Read the model definition and answer for the solid it produces. Units are mm, in the model's axes. Face numbers are marked on the shaded views. A direction names the side the tool comes from. Give positions to 0.01 mm unless a question says otherwise; leave off trailing zeros. Order: outer loops, then holes, each group sorted by start corner. A loop starts at its lowest first (then second) coordinate and runs counter-clockwise, first axis right, second up. Notation, with made-up numbers: (13.25, 6) -> (41.25, 6) arc R8 cw to (41.25, 15) -> close; hole circle Ø5 at (36, -33.75). An arc over 180 degrees is marked (long way). One line per item, written item: value. Start each with the question number.
from build123d import *

# Parameters (mm, degrees)
SKETCH_1_W      = 32
SKETCH_1_H      = 20
SKETCH_1_R      = 1.5
EXTRUDE_1_DEPTH = 1.6
SKETCH_2_W      = 6.5
SKETCH_2_H      = 6.5
EXTRUDE_2_DEPTH = 5
SKETCH_3_R      = 9.5
EXTRUDE_3_DEPTH = 16.5


with BuildPart() as part:
    # 草图1 → 凸台-拉伸1 (new body)
    with BuildSketch(Plane(origin=(0, 0, 0), x_dir=(1, 0, 0), z_dir=(0, 1, 0))):
        Rectangle(SKETCH_1_W, SKETCH_1_H)
        with Locations(Location((-13.5, 7.5, 0), (0, 0, 270))):
            Circle(SKETCH_1_R, mode=Mode.SUBTRACT)
        with Locations(Location((13.5, 7.5, 0), (0, 0, 270))):
            Circle(SKETCH_1_R, mode=Mode.SUBTRACT)
        with Locations(Location((-13.5, -7.5, 0), (0, 0, 270))):
            Circle(SKETCH_1_R, mode=Mode.SUBTRACT)
        with Locations(Location((13.5, -7.5, 0), (0, 0, 270))):
            Circle(SKETCH_1_R, mode=Mode.SUBTRACT)
    extrude(amount=EXTRUDE_1_DEPTH)

    # 草图2 → 凸台-拉伸2 (add)
    with BuildSketch(Plane(origin=(0, 0, 0), x_dir=(1, 0, 0), z_dir=(0, 1, 0))):
        with Locations((7.75, -6.25)):
            Rectangle(SKETCH_2_W, SKETCH_2_H)
    extrude(amount=-EXTRUDE_2_DEPTH)

    # 草图3 → 凸台-拉伸3 (add)
    with BuildSketch(Plane(origin=(0, 0, 0), x_dir=(1, 0, 0), z_dir=(0, 1, 0))):
        with Locations(Location((-5, 0, 0), (0, 0, 270))):
            Circle(SKETCH_3_R)
    extrude(amount=EXTRUDE_3_DEPTH)

    # 草图4 → 切除-旋转2 (revolve, cut)
    with BuildSketch(Plane.XY):
        Polygon((-0.3, 16.5), (0.5, 16.5), (4.5, 16.5), (4.5, 6.5), (3, 6.5), (0.766666667, 15.433333333), align=None)
    revolve(axis=Axis((-5, -983.5, 0), (0, 1, 0)), mode=Mode.SUBTRACT)


solid = part.part
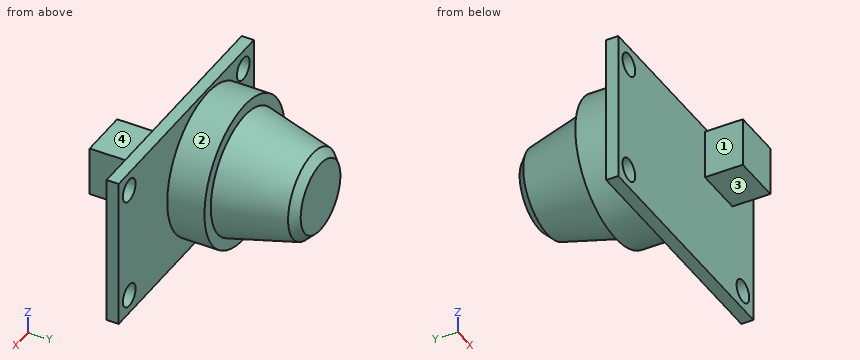
Item 1: Find section D-D on x = -5. Write down the section's boundary in (y, z).
Item 2: Find the intervals of material crossed by line 1 (X direction, y = 0.8, z = -7.5); line 2 (Z direction, x = 14, y = 1.5); line 3 (Y direction, x = -13, z = -5), in increasing order. Write a range as from..to.
Item 3: Flat-ended cylindrical pins translate along their axes: pin 1 (5 mm diameter, centred on x = 13.5, z = -7.5, fed in from -Y); pin 2 (2.5 mm diameter, centred on x = -13.5, z = 7.5, fed in from -Y); pin 3 (5.5 mm diameter, centred on y = -1.5, z = 7, fed in from -X); pin 4 (3 mm diameter, centred on x = -12.5, y = 6.5, fed in from -Z). Find the tip coordinate at first contact, or state that the pin passes through.
Item 4: Find section B-B on z = 0. Write down the section's boundary in (x, y).
Item 5: Find section C-C on y = 1. Write down the section's boundary in (x, z).
Item 6: A tool of negligible diameter and unlimited length cuts with its end or side. For the marked faces 1, 2, 3 and 4, from which of +Z, -Z, +X, -X, +Y, -Y can it reach the whole face along a straight path? Write none if from no direction.
Item 7: Find section A-A on x = 13.5. Write down the section's boundary in (y, z), then the cut area to 3 significant figures.
Checks:
1. outline: (0, -10) -> (1.6, -10) -> (1.6, -9.5) -> (6.5, -9.5) -> (6.5, -8) -> (15.43, -5.77) -> (16.5, -4.7) -> (16.5, 4.7) -> (15.43, 5.77) -> (6.5, 8) -> (6.5, 9.5) -> (1.6, 9.5) -> (1.6, 10) -> (0, 10) -> close
2. line 1: -16..-15, -12..12, 15..16
2. line 2: -10..-8.91, -6.09..6.09, 8.91..10
2. line 3: 0..6.5
3. pin 1: y = 0
3. pin 2: through
3. pin 3: x = -16
3. pin 4: z = -7.37
4. outline: (-16, 0) -> (16, 0) -> (16, 1.6) -> (4.5, 1.6) -> (4.5, 6.5) -> (3, 6.5) -> (0.77, 15.43) -> (-0.3, 16.5) -> (-9.7, 16.5) -> (-10.77, 15.43) -> (-13, 6.5) -> (-14.5, 6.5) -> (-14.5, 1.6) -> (-16, 1.6) -> close
5. outline: (-16, -10) -> (16, -10) -> (16, 10) -> (-16, 10) -> close; hole circle Ø3 at (-13.5, -7.5); hole circle Ø3 at (-13.5, 7.5); hole circle Ø3 at (13.5, -7.5); hole circle Ø3 at (13.5, 7.5)
6. face 1: +Z, -Z, -X, -Y
6. face 2: +Y
6. face 3: -Z, +X, -X, -Y
6. face 4: +Z, +X, -X, -Y
7. outline: (0, -10) -> (1.6, -10) -> (1.6, -9) -> (0, -9) -> close; (0, -6) -> (1.6, -6) -> (1.6, 6) -> (0, 6) -> close; (0, 9) -> (1.6, 9) -> (1.6, 10) -> (0, 10) -> close
7. area: 22.4 mm2
